Build history of the part. All positions in model axes, mm. Face numbers are marked on the shaded views. A direction names the side the tool comes from. Coordinates: 2 decimals unless noted, no trailing zeros. Loops run counter-clockwise (first coordinate to the right, second up) from the corner with the lowest first, then second, coordinate; pieces in that order, holes last. Notation, with made-up numbers: (44, 24) - (66, 24) arc R29 cw to (66, 59) - close; hole circle Ø2 at (0, 21). An arc over 180 degrees is marked (long way). One line per item, written item: value.
```python
from build123d import *

# Parameters (mm, degrees)
SKIZZE1_W                       = 150
SKIZZE1_H                       = 100
AUFSATZ_LINEAR_AUSTRAGEN1_DEPTH = 50
SKIZZE2_W                       = 100
SKIZZE2_H                       = 80
SCHNITT_LINEAR_AUSTRAGEN1_DEPTH = 5
SKIZZE3_W                       = 50
SKIZZE3_H                       = 50
AUFSATZ_LINEAR_AUSTRAGEN2_DEPTH = 2.5
SKIZZE4_R                       = 5
SCHNITT_LINEAR_AUSTRAGEN2_DEPTH = 10
SKIZZE5_W                       = 10
SKIZZE5_H                       = 100
SCHNITT_LINEAR_AUSTRAGEN3_DEPTH = 40
SKIZZE6_R                       = 5
SCHNITT_LINEAR_AUSTRAGEN4_DEPTH = 40


with BuildPart() as part:
    # Skizze1 → Aufsatz-Linear austragen1 (new body)
    with BuildSketch(Plane(origin=(0, 0, 0), x_dir=(0, 0, -1), z_dir=(1, 0, 0))):
        with Locations((-31.954225352, -9.463028169)):
            Rectangle(SKIZZE1_W, SKIZZE1_H)
    extrude(amount=AUFSATZ_LINEAR_AUSTRAGEN1_DEPTH)

    # Skizze2 → Schnitt-Linear austragen1 (cut)
    with BuildSketch(Plane(origin=(50, 0, 0), x_dir=(0, 0, -1), z_dir=(1, 0, 0))):
        with Locations((-6.954225352, -19.463028169)):
            Rectangle(SKIZZE2_W, SKIZZE2_H)
    extrude(amount=-SCHNITT_LINEAR_AUSTRAGEN1_DEPTH, mode=Mode.SUBTRACT)

    # Skizze3 → Aufsatz-Linear austragen2 (add)
    with BuildSketch(Plane(origin=(45, 0, 0), x_dir=(0, 0, -1), z_dir=(1, 0, 0))):
        with Locations((18.045774648, -19.463028169)):
            Rectangle(SKIZZE3_W, SKIZZE3_H)
    extrude(amount=AUFSATZ_LINEAR_AUSTRAGEN2_DEPTH)

    # Skizze4 → Schnitt-Linear austragen2 (cut)
    with BuildSketch(Plane(origin=(47.5, 0, 0), x_dir=(0, 0, -1), z_dir=(1, 0, 0))):
        with Locations((33.045774648, -19.463028169)):
            Circle(SKIZZE4_R)
        with Locations((13.045774648, -19.463028169)):
            Circle(SKIZZE4_R)
    extrude(amount=-SCHNITT_LINEAR_AUSTRAGEN2_DEPTH, mode=Mode.SUBTRACT)

    # Skizze5 → Schnitt-Linear austragen3 (cut)
    with BuildSketch(Plane.XY.offset(106.954225352)):
        with Locations((5, -9.463028169)):
            Rectangle(SKIZZE5_W, SKIZZE5_H)
        with Locations((45, -9.463028169)):
            Rectangle(SKIZZE5_W, SKIZZE5_H)
    extrude(amount=-SCHNITT_LINEAR_AUSTRAGEN3_DEPTH, mode=Mode.SUBTRACT)

    # Skizze6 → Schnitt-Linear austragen4 (cut)
    with BuildSketch(Plane(origin=(40, 0, 0), x_dir=(0, 0, -1), z_dir=(1, 0, 0))):
        with Locations(Location((-86.954225352, -9.463028169, 0), (0, 0, 90))):
            Circle(SKIZZE6_R)
    extrude(amount=-SCHNITT_LINEAR_AUSTRAGEN4_DEPTH, mode=Mode.SUBTRACT)


solid = part.part
```
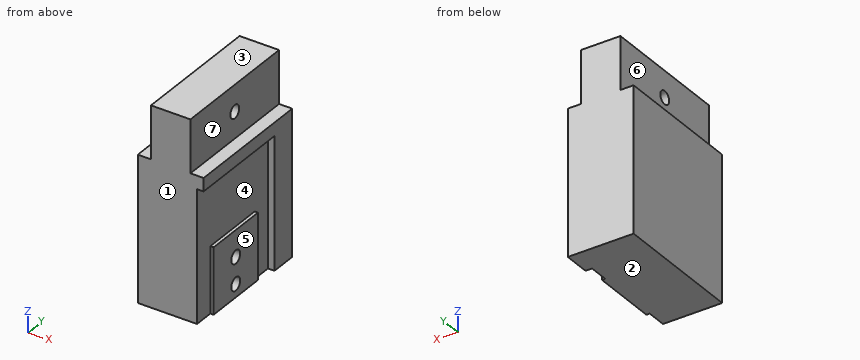
Item 1: Pull direction Z, two halves, no side cores. Call the marked faces 1, 2, 3 and 4: released by +Z, released by -Z, zero draft, split by the parting line, or undercut.
Check result:
face 1: zero draft
face 2: released by -Z
face 3: released by +Z
face 4: undercut
Item 2: Cut at B-B, the plane y = -12. Write the cut outline in (x, z), then the cut area to 3 significant figures.
Check result:
outline: (0, -43.05) - (47.5, -43.05) - (47.5, 6.95) - (45, 6.95) - (45, 56.95) - (50, 56.95) - (50, 66.95) - (40, 66.95) - (40, 82.65) - (10, 82.65) - (10, 66.95) - (0, 66.95) - close; (10, 91.26) - (40, 91.26) - (40, 106.95) - (10, 106.95) - close
area: 6,070 mm^2
Item 3: Drop flat-ended pins along their axis: P1, Ø1.2, axis at x = 46, z = -30, coming from the -Y side; P2, Ø1.2, axis at x = 46.5, y = -30.5, coming from the +Z side; P3, Ø11, axis at y = -20.5, z = -32.5, coming from the +X side. Give the stop position or say it passes through.
Check result:
P1: stops at y = -44.46
P2: stops at z = 66.95
P3: stops at x = 47.5
Item 4: Probe probe 1 along Z at (x, y) = (11, -9); probe 2 along Z at (x, y) = (4, 3.5); probe 3 along X at (y, z) = (-22, 50.5). List the from-to ranges inside material, lowest first. Write a range as from..to.
Check result:
probe 1: z = -43.05..81.98, 91.93..106.95
probe 2: z = -43.05..66.95
probe 3: x = 0..45
Item 5: Cut at A-A, the plane z = -21. Write the cut outline in (x, y), then the cut area to 4 significant figures.
Check result:
outline: (0, -59.46) - (45, -59.46) - (45, -44.46) - (47.5, -44.46) - (47.5, 5.54) - (45, 5.54) - (45, 20.54) - (50, 20.54) - (50, 40.54) - (0, 40.54) - close
area: 4,725 mm^2
Item 6: Cut at C-C, the plane y = -31. Write the cut outline in (x, z), then the cut area to 4 significant figures.
Check result:
outline: (0, -43.05) - (47.5, -43.05) - (47.5, 6.95) - (45, 6.95) - (45, 56.95) - (50, 56.95) - (50, 66.95) - (40, 66.95) - (40, 106.95) - (10, 106.95) - (10, 66.95) - (0, 66.95) - close
area: 6,325 mm^2
Item 7: Cut at D-D, the plane x = 8. Write the cut outline in (y, z).
Check result:
outline: (-59.46, -43.05) - (40.54, -43.05) - (40.54, 66.95) - (-59.46, 66.95) - close
Item 8: Tool access for the marked faces 5, 6 and 7: list every direction of +Z, -Z, +X, -X, +Y, -Y with a clear straight run to the whole face (end or side of a thin tool).
Check result:
face 5: -Z, +X, -Y
face 6: +Z, -X, +Y, -Y
face 7: +Z, +X, +Y, -Y
